Can you work these out from the model? Positions are in its coordinate system, mm. A direction names the side the tool comes from. Give positions to 0.01 mm unless a question says otherwise; leave off trailing zeros. Write each loop counter-clockwise with the first axis right and the second up, starting at its lowest first coordinate (ties: lowest second). Pieces come first, ordered by that corner, then holes. Notation, with made-up numbers: (20, -19) -> (34, -19) arc R13 cw to (34, 0) -> close; hole circle Ø8 at (15.5, 14). An arc over 180 degrees is marked (long way). One line per item, written item: value.
from build123d import *

# Parameters (mm, degrees)
F0_R     = 1.38938
F0_R_2   = 2.13995
F1_DEPTH = 6.35
F2_W     = 17.878901
F2_H     = 3.15336
F2_H_2   = 3.638602
F3_DEPTH = 38.101
F4_W     = 17.966992
F4_H     = 2.413
F5_DEPTH = 57.151
F6_R     = 1.524


with BuildPart() as f1:
    # F0 (on Top) → F1 (new body)
    with BuildSketch(Plane.XY):
        with BuildLine():
            ThreePointArc((-29.464, 0.889), (-28.534064, -1.356064), (-26.289, -2.286))
            Line((-26.289, -2.286), (-5.334, -2.286))
            ThreePointArc((-5.334, -2.286), (0.054154, -4.517846), (2.286, -9.906))
            Line((2.286, -9.906), (2.286, -49.911))
            ThreePointArc((2.286, -49.911), (3.215936, -52.156064), (5.461, -53.086))
            ThreePointArc((5.461, -53.086), (7.706064, -52.156064), (8.636, -49.911))
            Line((8.636, -49.911), (8.636, 4.064))
            Line((8.636, 4.064), (-26.289, 4.064))
            ThreePointArc((-26.289, 4.064), (-28.534064, 3.134064), (-29.464, 0.889))
        make_face()
        with Locations((5.461, -43.561)):
            Circle(F0_R, mode=Mode.SUBTRACT)
        with Locations((-21.7932, 0.889)):
            Circle(F0_R, mode=Mode.SUBTRACT)
        with Locations((4.572, 0)):
            Circle(F0_R_2, mode=Mode.SUBTRACT)
    extrude(amount=F1_DEPTH)

    # F2 (on face) → F3 (cut, through all)
    with BuildSketch(Plane.YZ.offset(8.636)):
        with Locations((-46.277451, 5.51368)):
            Rectangle(F2_W, F2_H)
        with Locations((-46.277451, 0.593699)):
            Rectangle(F2_W, F2_H_2)
    extrude(amount=-F3_DEPTH, mode=Mode.SUBTRACT)

    # F4 (on face) → F5 (cut, through all)
    with BuildSketch(Plane(origin=(0, 4.064, 0), x_dir=(-1, 0, 0), z_dir=(0, 1, 0))):
        with Locations((24.477496, 5.1435)):
            Rectangle(F4_W, F4_H)
        with Locations((24.477496, 1.2065)):
            Rectangle(F4_W, F4_H)
    extrude(amount=-F5_DEPTH, mode=Mode.SUBTRACT)

    # F6
    f6_edges = [f1.edges().sort_by_distance(p)[0] for p in [
        (-15.494, 0.889, 3.937),
        (-15.494, 0.889, 2.413),
        (5.461, -37.338, 3.937),
        (5.461, -37.338, 2.413),
    ]]
    fillet(f6_edges, radius=F6_R)


solid = f1.part
1) If we section it at D-D (x = -27): Write out the boundary of the cut face in (y, z), and give its area (3 significant figures).
Answer list:
outline: (-2.21, 2.41) -> (3.98, 2.41) -> (3.98, 3.94) -> (-2.21, 3.94) -> close
area: 9.43 mm^2
2) For faces 5 (the face through (6, -46, 2.413)), 6 (the face through (-23.2, 0.2, 2.413)), 7 (the face through (6, -46, 3.937)), 8 (the face through (-14, -2.286, 3)), 9 (the face through (-23.2, 0.2, 3.937)), which set-ups out of +Z, -Z, +X, -X, +Y, -Y let a thin tool reach every point of the face, with its end or its side?
Answer list:
face 5: -Z, +X, -X, -Y
face 6: -Z, -X, +Y, -Y
face 7: +Z, +X, -X, -Y
face 8: +Z, -Z, -X, -Y
face 9: +Z, -X, +Y, -Y
3) Will these pins go through, and if not, where does the flat tip stop? pin 1 (1.9 mm diameter, centred on x = 5, y = -45.5, fed in from -Z); pin 2 (5 mm diameter, centred on x = 5, y = -46, fed in from +Z); pin 3 (1 mm diameter, centred on x = 6, z = 0.5, fed in from -Y).
Answer list:
pin 1: stops at z = 2.41
pin 2: stops at z = 3.94
pin 3: stops at y = -37.34
4) If we section it at B-B (z = 4.5): Write out the boundary of the cut face in (x, y).
Answer list:
outline: (-15.84, -2.29) -> (-5.33, -2.29) arc R7.62 cw to (2.29, -9.91) -> (2.29, -37.68) -> (8.64, -37.68) -> (8.64, 4.06) -> (-15.84, 4.06) -> close; hole circle Ø4.28 at (4.57, 0)
5) If we section it at C-C (y = -19): Write out the boundary of the cut face in (x, z), and give its area (3 significant figures).
Answer list:
outline: (2.29, 0) -> (8.64, 0) -> (8.64, 6.35) -> (2.29, 6.35) -> close
area: 40.3 mm^2
6) We'd pull the mould along X, two halves only. Please class faces 1 (the face through (-15.952, 0.845, 1.978)), 2 (the face through (2.434, 0.094, 3.131)), 3 (the face through (5.28, -42.183, 3.164)), 4 (the face through (5.42, -37.77, 1.95)): released by +X, released by -X, zero draft, split by the parting line, or undercut.
Answer list:
face 1: released by -X
face 2: undercut
face 3: undercut
face 4: zero draft
7) I need wall thicknesses on L1, parallel to Y at x = -9, z = 4; L2, parallel to Y at x = 5, z = 0.5; L3, parallel to Y at x = 5, z = 3.5. Which ranges of each line are inside material? Lowest first, please.
Answer list:
L1: y = -2.29 to 4.06
L2: y = -37.34 to -2.1, 2.1 to 4.06
L3: y = -53.05 to -44.87, -42.25 to -2.1, 2.1 to 4.06
8) If we section it at A-A (x = -21): Write out the boundary of the cut face in (y, z).
Answer list:
outline: (-2.29, 2.41) -> (-0.25, 2.41) -> (-0.25, 3.94) -> (-2.29, 3.94) -> close; (2.03, 2.41) -> (4.06, 2.41) -> (4.06, 3.94) -> (2.03, 3.94) -> close
